Design review of the part built by this model. Coordinates are the model's own, in mm. Coordinates: 2 decimals unless noted, no trailing zeros. Write each loop counter-clockwise with the first axis right and the second up, starting at its lowest first coordinate (ties: lowest second). Pieces come first, ordered by that corner, then holes.
Q1. Take a section at B-B, the plane y = -4.5. Write out the cut boundary in (x, z), plus the area to 3 significant figures.
Q2. Take a section at C-C, the plane x = -15.5. Write out the cut boundary in (y, z).
Q3. Take a section at A-A, the plane z = 2.25. Write out the cut boundary in (x, y), plus the area to 3 significant figures.
Q4. For L1, parallel to Z at x = 56, y = 44; L2, parallel to X at y = 50, z = 1.75; L3, parallel to Y at x = 31.5, z = 3.25, list the stretches that pass through material, from the lowest coordinate up.
Q5. For pin 1 Ø4 at (x, z) = (23, 5.5) entering from -Y; pin 2 Ø3 at (x, y) = (45, 81.5) entering from +Z; pin 3 Ø6 at (x, y) = (-50.5, 6) entering from +Z, all flat-tipped, find the tip position at first contact; note any pin that passes through.
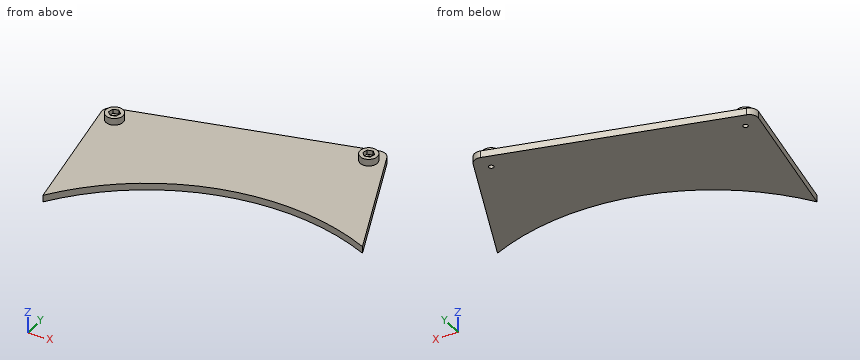
Autodesk Inventor part; units mm, degrees
ref_plane "YZ Plane" through (0, 0, 0) normal (1, 0, 0) x (0, 1, 0)
ref_plane "XZ Plane" through (0, 0, 0) normal (0, 1, 0) x (-1, 0, 0)
ref_plane "XY Plane" through (0, 0, 0) normal (0, 0, 1) x (1, 0, 0)
ref_plane "Płaszczyzna konstrukcyjna1" through (0, 0, 0) normal (0, 0, 1) x (1, 0, 0)
sketch "Szkic1" plane through (0, 0, 0) normal (0, 0, 1) x (1, 0, 0)
  line L0 (-77.9596, -24.5647) -> (-89.3248, 51.2994)
  arc A0 (-85.674, 56.8699) -> (-89.3248, 51.2994) centre (-84.3799, 52.0402) ccw
  line L1 (-85.674, 56.8699) -> (45.761, 92.0878)
  arc A1 (51.7078, 89.089) -> (45.761, 92.0878) centre (47.0551, 87.2581) ccw
  line L2 (51.7078, 89.089) -> (79.7973, 17.7061)
  circle A2 centre (27.7277, -103.4811) radius 131.9
  line L3 (-77.9596, -24.5647) -> (-89.3248, 51.2994)
  line L4 (79.7973, 17.7061) -> (51.7078, 89.089)
  arc A3 (79.7973, 17.7061) -> (-77.9596, -24.5647) centre (27.7277, -103.4811) ccw
  arc A4 (-85.674, 56.8699) -> (-89.3248, 51.2994) centre (-84.3799, 52.0402) ccw
  arc A5 (51.7078, 89.089) -> (45.761, 92.0878) centre (47.0551, 87.2581) ccw
  line L5 (-85.674, 56.8699) -> (45.761, 92.0878)
  point P0 (0, 0)
extrude "Wyciągnięcie proste1" add sketch "Szkic1" along normal blind 4 contours L0 A0 L1 A1 L2 A2
sketch "Szkic2" plane through (0, 0, 4) normal (0, 0, 1) x (1, 0, 0)
  circle A0 centre (-80.4123, 48.9622) radius 5
  line L0 (-37.9291, 141.5533) -> (24.1284, -90.0484) construction
  line L1 (45.761, 92.0878) -> (-85.674, 56.8699) construction
  circle A1 centre (45.158, 82.6087) radius 5
  point P0 (0, 0)
  dimension "d2" = 10
  dimension "d3" = 65
  dimension "d4" = 9
extrude "Wyciągnięcie proste2" add sketch "Szkic2" along normal blind 4
sketch "Szkic3" plane through (45.158, 82.6087, 8) normal (0, 0, 1) x (1, 0, 0)
  circle A0 centre (0, 0) radius 5
  circle A1 centre (-125.5704, -33.6465) radius 5
  line L0 (-124.7784, -30.6908) -> (-122.6147, -32.8545)
  line L1 (-122.6147, -32.8545) -> (-123.4066, -35.8102)
  line L2 (-123.4066, -35.8102) -> (-126.3623, -36.6022)
  line L3 (-126.3623, -36.6022) -> (-128.526, -34.4385)
  line L4 (-128.526, -34.4385) -> (-127.7341, -31.4828)
  line L5 (-127.7341, -31.4828) -> (-124.7784, -30.6908)
  line L6 (0.792, 2.9557) -> (2.9557, 0.792)
  line L7 (2.9557, 0.792) -> (2.1637, -2.1637)
  line L8 (2.1637, -2.1637) -> (-0.792, -2.9557)
  line L9 (-0.792, -2.9557) -> (-2.9557, -0.792)
  line L10 (-2.9557, -0.792) -> (-2.1637, 2.1637)
  line L11 (-2.1637, 2.1637) -> (0.792, 2.9557)
  line L12 (0.6029, 9.479) -> (-130.832, -25.7389)
  point P0 (-45.158, -82.6087)
  dimension "d7" = 5.3
  dimension "d8" = 5.3
extrude "Wyciągnięcie proste3" cut sketch "Szkic3" against normal blind 2.5 contours L0 L1 L2 L3 L4 L5 | L6 L7 L8 L9 L10 L11
sketch "Szkic4" plane through (45.158, 82.6087, 5.5) normal (0, 0, 1) x (1, 0, 0)
  circle A0 centre (0, 0) radius 5
  circle A1 centre (-125.5704, -33.6465) radius 5
  circle A2 centre (0, 0) radius 1.35
  circle A3 centre (-125.5704, -33.6465) radius 1.35
  point P0 (-45.158, -82.6087)
  dimension "d11" = 2.7
  dimension "d12" = 2.7
extrude "Wyciągnięcie proste4" cut sketch "Szkic4" against normal up to next contours A2 | A3
equation "\"d8\" = d7"
equation "\"d12\" = d11"
properties part number "housing_undercover"
Responses:
1. outline: (-80.97, 0) - (-59.45, 0) - (-59.45, 4) - (-80.97, 4) - close
1. area: 86.1 mm2
2. outline: (21.13, 0) - (75.67, 0) - (75.67, 4) - (21.13, 4) - close
3. outline: (-89.32, 51.3) - (-77.96, -24.56) arc R131.9 cw to (79.8, 17.71) - (51.71, 89.09) arc R5 ccw to (45.76, 92.09) - (-85.67, 56.87) arc R5 ccw to start; hole circle Ø2.7 at (-80.41, 48.96); hole circle Ø2.7 at (45.16, 82.61)
3. area: 9,260 mm2
4. L1: z = 0 to 4
4. L2: x = -89.13 to -81.28, -79.55 to 67.09
4. L3: y = 28.36 to 88.27
5. pin 1: stops at y = 28.28
5. pin 2: stops at z = 5.5
5. pin 3: stops at z = 4
